Geometry check sheet. Reference: drawing and pictorial views, mm from the part's lowest x, y, z. A direction names the side the tool comes from. Round coordinates to 2 decimals unless told otherwise and drop trailing zeros. Write each loop counter-clockwise with the first axis right and the second up, starting at its lowest first coordinate (ties: lowest second). Pieces come first, ordered by that corner, then holes. Notation, with made-up numbers: M -5,-26 L -1,-26 A15 cw -1,-12 Z; hole C -12,9.25 d1. An arc over 180 degrees is marked long. Answer in a Markdown table with one row per item.
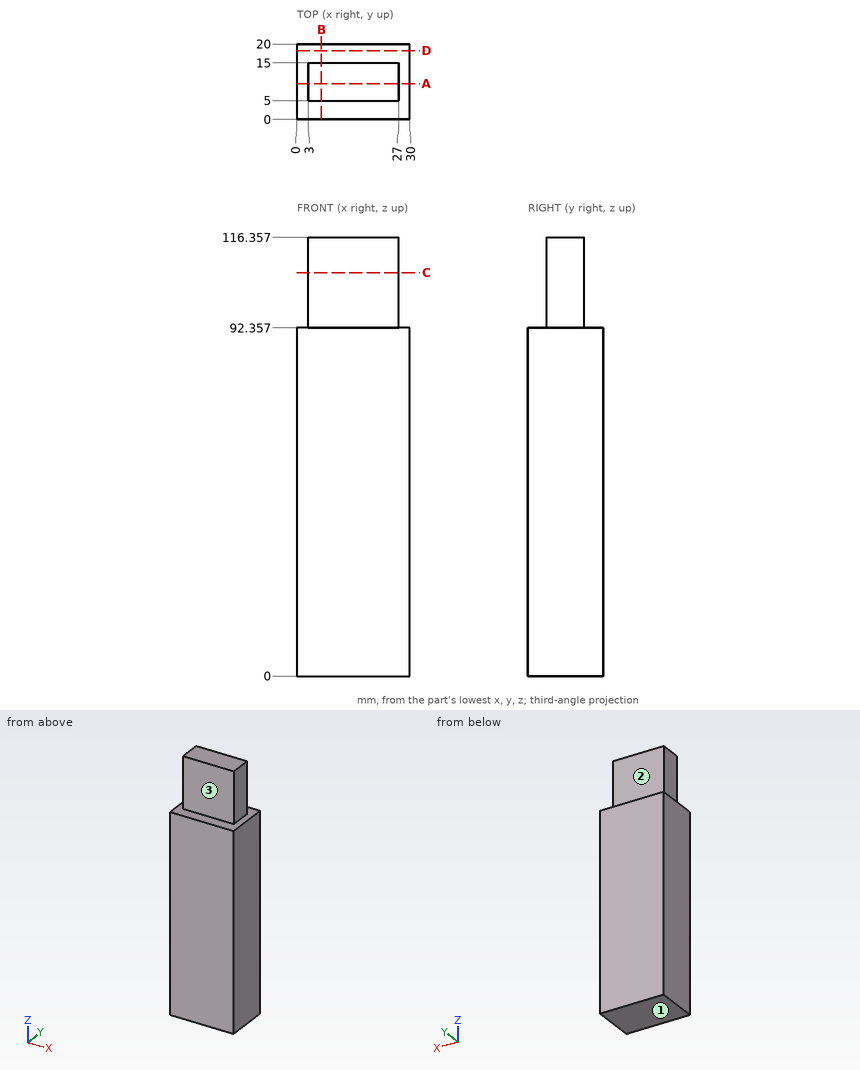
1. Scan lines: L1, parallel to Z at x = 28, y = 10.5; L2, parallel to X at y = 14.5, z = 107; L3, parallel to Y at x = 3.25, z = 97.5. Record each from-to range of solid material in increasing order.
Found:
| item | result |
|---|---|
| L1 | z = 0 to 92.36 |
| L2 | x = 3 to 27 |
| L3 | y = 5 to 15 |
2. Section check A-A, the plane y = 9.5. Record the cut outline in (x, z).
Found:
| item | result |
|---|---|
| outline | M 0,0 L 30,0 L 30,92.36 L 27,92.36 L 27,116.36 L 3,116.36 L 3,92.36 L 0,92.36 Z |
3. Section check B-B, the plane x = 6.5. Record the cut outline in (y, z).
Found:
| item | result |
|---|---|
| outline | M 0,0 L 20,0 L 20,92.36 L 15,92.36 L 15,116.36 L 5,116.36 L 5,92.36 L 0,92.36 Z |
4. Section check C-C, the plane z = 107. Record the cut outline in (x, y).
Found:
| item | result |
|---|---|
| outline | M 3,5 L 27,5 L 27,15 L 3,15 Z |
5. Access from +Z, -Z, +X, -X, +Y, -Y to the whole of each face (thin tool, end or side, straight path). Record for the marked faces 1, 2 and 3.
Found:
| item | result |
|---|---|
| face 1 | -Z, +X, -X, +Y, -Y |
| face 2 | +Z, +X, -X, +Y |
| face 3 | +Z, +X, -X, -Y |
6. Section check D-D, the plane y = 18.25. Record the cut outline in (x, z), and give its area (3 significant figures).
Found:
| item | result |
|---|---|
| outline | M 0,0 L 30,0 L 30,92.36 L 0,92.36 Z |
| area | 2,770 mm2 |
7. Go/stop test with flat-tipped pins: pin 1 (5 mm diameter, centred on y = 10, z = 108, fed in from +X); pin 2 (7 mm diameter, centred on x = 18, z = 98.5, fed in from +Y); pin 3 (11 mm diameter, centred on y = 10, z = 99, fed in from -X). Record where each tip stops, or that it passes through.
Found:
| item | result |
|---|---|
| pin 1 | stops at x = 27 |
| pin 2 | stops at y = 15 |
| pin 3 | stops at x = 3 |
